Model file for the job. Use its own axes, mm. A direction names the side the tool comes from. Round coordinates to 2 decimals unless told otherwise and drop trailing zeros. Write each loop counter-clockwise with the first axis right and the second up, starting at its lowest first coordinate (ties: lowest second). Pieces come first, ordered by that corner, then holes. Notation, with made-up numbers: (-16, -23) - (33, -23) arc R14 cw to (33, -4) - close; hole circle Ø10 at (-2, 57). An arc over 180 degrees is marked (long way). Answer as a JSON object with one key per item and string values. Group by question number.
from build123d import *

# Parameters (mm, degrees)
SKETCH1_R           = 1
SKETCH1_W           = 24
SKETCH1_H           = 12
BOSS_EXTRUDE2_DEPTH = 10
CHAMFER1_SIZE       = 5
SKETCH3_R           = 1.25
CUT_EXTRUDE1_DEPTH  = 12
BOSS_EXTRUDE3_DEPTH = 10
CHAMFER2_SIZE       = 5


with BuildPart() as part:
    # Sketch1 → Boss-Extrude2 (new body)
    with BuildSketch(Plane(origin=(0, 0, 0), x_dir=(1, 0, 0), z_dir=(0, 1, 0))):
        Polygon((-18.962264151, -7.55754717), (19.037735849, -7.55754717), (19.037735849, 4.79245283), (19.037735849, 16.79245283), (-18.962264151, 16.79245283), (-18.962264151, 4.79245283), align=None)
        with Locations(Location((-13.962264151, 4.79245283, 0), (0, 0, 270))):
            Circle(SKETCH1_R, mode=Mode.SUBTRACT)
        with Locations(Location((14.037735849, 4.79245283, 0), (0, 0, 270))):
            Circle(SKETCH1_R, mode=Mode.SUBTRACT)
        with Locations((0.037735849, 4.79245283)):
            Rectangle(SKETCH1_W, SKETCH1_H, mode=Mode.SUBTRACT)
    extrude(amount=BOSS_EXTRUDE2_DEPTH)

    # Chamfer1
    chamfer1_edges = [part.edges().sort_by_distance(p)[0] for p in [
        (19.037735849, 5, 7.55754717),
        (-18.962264151, 5, 7.55754717),
        (-18.962264151, 5, -16.79245283),
        (19.037735849, 5, -16.79245283),
    ]]
    chamfer(chamfer1_edges, length=CHAMFER1_SIZE)

    # Sketch3 → Cut-Extrude1 (cut)
    with BuildSketch(Plane.XY.offset(7.55754717)):
        with Locations((-7.712264151, 5)):
            Circle(SKETCH3_R)
        with Locations((7.787735849, 5)):
            Circle(SKETCH3_R)
    extrude(amount=-CUT_EXTRUDE1_DEPTH, mode=Mode.SUBTRACT)

    # Sketch4 → Boss-Extrude3 (add)
    with BuildSketch(Plane(origin=(0, 10, 0), x_dir=(1, 0, 0), z_dir=(0, 1, 0))):
        Polygon((-13.962264151, -7.55754717), (-13.962264151, -12.55754717), (-18.962264151, -12.55754717), (-18.962264151, -2.55754717), (-13.962264151, -0.983393269), align=None)
    extrude(amount=-BOSS_EXTRUDE3_DEPTH)

    # Chamfer2
    chamfer2_edges = [part.edges().sort_by_distance(p)[0] for p in [
        (-18.962264151, 5, 12.55754717),
    ]]
    chamfer(chamfer2_edges, length=CHAMFER2_SIZE - 0.0001)  # a hair under: the kernel refuses the full size


solid = part.part
(1) Slice it at B-B (z = -1.75). Write the cut outline in (x, y), then the cut area to 3 significant figures.
(2) Pull direction X, two halves, no side cores. Call faces 5 (the flat face through (0, 10, 4)), 6 (the flat face through (16.573, 4.93, 5.023)), 7 (the cylindrical face through (6.796, 4.239, 4.427)), 8 (the flat face through (-18.962, 5, -2)): pulls with the +X half, pulls with the -X half, needs draft (parallel to the pull), parting line crosses it, or undercut.
(3) Drill centre lines: line 1 (Z direction, x = -7.5, y = 8); line 2 (X direction, y = 4, z = -2.75); line 3 (X direction, y = 4.5, z = -4.25). Where is each one in solid material? Low to high. Write a range as from..to.
(4) 3-axis set-ups, long thin cutter, end or side, ignore diameter. For faces 1 (the flat face through (0, 5, -10.792)), 2 (the flat face through (-16.5, 5.07, 10.02)), 3 (the cylindrical face through (-8.704, 4.239, 4.427)), 4 (the flat face through (-13.962, 5, 10)): which of +Z, -Z, +X, -X, +Y, -Y reach the whole face in a straight line?
(5) Slice it at C-C (x = 1). Write the cut outline in (y, z), then the cut area to 4 significant figures.
(6) Slice it at A-A (y = 5). Count the separate pieces of the cut face and the enclosed holes in it, then the cut area to 3 significant figures.
(7) Flat gauge pins, fed straight in: pin 1 (2.5 mm diameter, centred on y = 4.5, z = 11, fed in from +X); pin 2 (5 mm diameter, centred on x = 13.5, y = 3, fed in from +Z). Where does each tip first touch, or does it go through?
Answer:
{
 "1": {"outline": "(-18.96, 0) - (-11.96, 0) - (-11.96, 10) - (-18.96, 10) - close; (12.04, 0) - (19.04, 0) - (19.04, 10) - (12.04, 10) - close", "area": "140 mm²"},
 "2": {"face 5": "needs draft", "face 6": "pulls with the +X half", "face 7": "undercut", "face 8": "pulls with the -X half"},
 "3": {"line 1": "-16.79..-10.79, 1.21..7.56", "line 2": "-18.96..-11.96, 12.04..19.04", "line 3": "-18.96..-14.8, -13.12..-11.96, 12.04..13.2, 14.88..19.04"},
 "4": {"face 1": "+Y, -Y", "face 2": "+Z, -X, +Y, -Y", "face 3": "+Z", "face 4": "+Z, +X, +Y, -Y"},
 "5": {"outline": "(0, -16.79) - (10, -16.79) - (10, -10.79) - (0, -10.79) - close; (0, 1.21) - (10, 1.21) - (10, 7.56) - (0, 7.56) - close", "area": "123.5 mm²"},
 "6": {"separate pieces": "2", "enclosed holes": "2", "area": "574 mm²"},
 "7": {"pin 1": "x = -13.96", "pin 2": "z = 7.56"}
}
